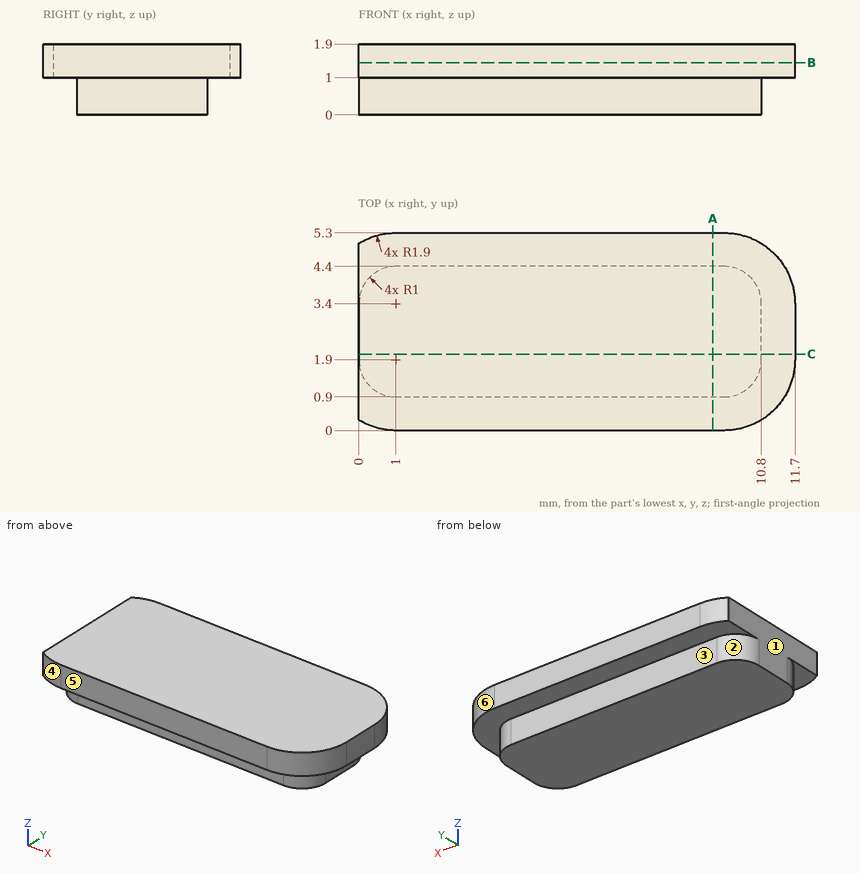
The figure shows three views and two pictorial views of one solid part (mm, origin at its lowest corner). Answer the questions. A direction names the side the tool comes from. Round coordinates to 2 decimals unless told otherwise and drop trailing zeros. Loops run counter-clockwise (first coordinate to the right, second up) from the corner with the lowest first, then second, coordinate; pieces in that order, holes last. Notation, with made-up numbers: (57.25, -1) - (87.25, -1) arc R16 cw to (87.25, 29) - close; hole circle Ø9 at (-8, 77.25). An arc over 180 degrees is marked (long way). One line per question, with ' | ' between items. Start each with the question number.
Q1. Section C-C on y = 2.05 is taken. Give the vertices of the cut face in (x, z).
Q2. Section B-B on z = 1.4 is taken. Give the vertices of the cut face in (x, y), plus the area to 3 significant figures.
Q3. For a pull along X with two mould halves and no side action, classify the marked faces 4, 5 and 6 as +X half, -X half, draft (parallel to the pull), parting line (faces both ways), or undercut.
Q4. A flat-ended cylindrical pin translates along its axis: pin 1 (0.5 mm diameter, centred on x = 4, z = 0.5, fed in from -Y). Find the tip coordinate at first contact, or state that the pin passes through.
Q5. Find the intervals of material crossed by L1, parallel to Y at x = 3.75, z = 0.95; L2, parallel to X at y = 1.95, z = 0.7; L3, parallel to Z at x = 10.75, y = 3.8, in increasing order.
Q6. Section A-A on x = 9.5 is taken. Give the vertices of the cut face in (y, z), plus the area to 3 significant figures.
Q7. For the marked faces 1, 2 and 3, determine the directions among +Z, -Z, +X, -X, +Y, -Y from which every point of the face is accessible in a straight line to the end or side of a thin tool.
Established:
1) outline: (0, 0) - (10.8, 0) - (10.8, 1) - (11.7, 1) - (11.7, 1.9) - (0, 1.9) - close
2) outline: (0, 0.28) arc R1.9 ccw to (1, 0) - (9.8, 0) arc R1.9 ccw to (11.7, 1.9) - (11.7, 3.4) arc R1.9 ccw to (9.8, 5.3) - (1, 5.3) arc R1.9 ccw to (0, 5.02) - close | area: 60.3 mm²
3) face 4: -X half | face 5: draft | face 6: +X half
4) pin 1: y = 0.9
5) L1: 0.9 to 4.4 | L2: 0 to 10.8 | L3: 1 to 1.9
6) outline: (0, 1) - (0.9, 1) - (0.9, 0) - (4.4, 0) - (4.4, 1) - (5.3, 1) - (5.3, 1.9) - (0, 1.9) - close | area: 8.27 mm²
7) face 1: +Z, -Z, -X, +Y, -Y | face 2: -Z, -X, +Y | face 3: -Z, +X, -X, +Y
